The listing builds one solid part. Answer for the finished solid, in the listing's coordinates (mm). A direction names the side the tool comes from. Round coordinates to 2 decimals unless told otherwise and drop trailing zeros. Write each loop counter-clockwise with the first axis right and the second up, starting at its lowest first coordinate (ties: lowest second). Pieces come first, ordered by that corner, then holes. Notation, with made-up numbers: M 82.5,-3 L 135.5,-3 A16 cw 135.5,21 Z; hole C 13.5,38 d6. An arc over 180 degrees is marked long. Put each result on its own line as item: value. Start each with the question number.
Autodesk Inventor part; units mm, degrees
ref_plane "YZ Plane" through (0, 0, 0) normal (1, 0, 0) x (0, 1, 0)
ref_plane "XZ Plane" through (0, 0, 0) normal (0, 1, 0) x (-1, 0, 0)
ref_plane "XY Plane" through (0, 0, 0) normal (0, 0, 1) x (1, 0, 0)
sketch "Sketch9" plane through (0, 0, 0) normal (0, 1, 0) x (-1, 0, 0)
  line L0 (15, 15) -> (-15, 15)
  line L1 (-15, 15) -> (-15, -15)
  line L2 (-15, -15) -> (15, -15)
  line L3 (15, -15) -> (15, 15)
  line L4 (15, 15) -> (-15, -15) construction
  line L5 (-15, 15) -> (15, -15) construction
  line L6 (-13, 13) -> (13, 13)
  line L7 (13, 13) -> (13, -13)
  line L8 (13, -13) -> (-13, -13)
  line L9 (-13, -13) -> (-13, 13)
  point P0 (0, 0)
  dimension "d172" = 30
  dimension "d173" = 30
  dimension "d174" = 2
extrude "Extrusion3" add sketch "Sketch9" against normal blind 250
sketch "Sketch10" plane through (0, 0, 0) normal (1, 0, 0) x (0, 1, 0)
  line L0 (0, 15) -> (0, -15) construction
  line L1 (0, 15) -> (-250, 15) construction
  line L2 (0, -15) -> (-250, -15) construction
  line L3 (-58.5, 8.5) -> (-41.5, 8.5)
  line L4 (-41.5, 8.5) -> (-41.5, -8.5)
  line L5 (-41.5, -8.5) -> (-58.5, -8.5)
  line L6 (-58.5, -8.5) -> (-58.5, 8.5)
  line L7 (-58.5, 8.5) -> (-41.5, -8.5) construction
  line L8 (-41.5, 8.5) -> (-58.5, -8.5) construction
  line L9 (0, 0) -> (30, 0)
  circle A0 centre (-50, 0) radius 8.5
  dimension "d177" = 17
  dimension "d178" = 17
  dimension "d181" = 30
  dimension "d182" = 80
extrude "Extrusion4" cut sketch "Sketch10" along normal through all contours A0
pattern_linear "Rectangular Pattern4" count 4 spacing 68 along (0, -1, 0) of "Extrusion4"
properties part number "PRS 1662 FDS 1000 way tube 4_D940" material "Stainless Steel"
Item 1: Section D-D (y = -118) is taken. Give the vertices of the cut face in (x, z), and give its area (3 significant figures).
Item 2: Section B-B (z = 0) is taken. Give the vertices of the cut face in (x, y), and give its area (3 significant figures).
Item 3: Section A-A (x = 3.5) is taken. Give the vertices of the cut face in (y, z).
Item 4: Which of the six approach directions +Z, -Z, +X, -X, +Y, -Y give full straight-line access (tool end or side, diameter ignored) to faces 4 (the flat face through (-13.3, -250, -1)), 5 (the flat face through (0, -123, -13)), 6 (the cylindrical face through (13.99, -109.89, -2.55))?
Item 5: Section C-C (y = -68) is taken. Give the vertices of the cut face in (x, z), and give its area (3 significant figures).
Item 6: A flat-ended cylindrical pin translates along its axis: pin 1 (13.5 mm diameter, centred on y = -118, z = 0, fed in from +X). Find the tip coordinate at first contact, or state that the pin passes through.
Item 7: Determine the mould class of faces 1 (the cylindrical face through (14, -245.5, 0.1)), 2 (the flat face through (15, -123.3, 6.9)), 3 (the flat face through (0, -123, 15)) for opening direction Z: released by +Z, released by -Z, zero draft, split by the parting line, or undercut.
Item 8: Consider line 1 along Y through (x, z) = (14.3, 0); line 2 along Z through (x, y) = (14.6, -50); line 3 along Z through (x, y) = (-8.5, -231.5). Determine where each line is inside the solid, lowest interval first. Write a range as [from, to].
Output values:
1. outline: M -15,-15 L 15,-15 L 15,-8.5 L 13,-8.5 L 13,-13 L -13,-13 L -13,13 L 13,13 L 13,8.5 L 15,8.5 L 15,15 L -15,15 Z
1. area: 190 mm^2
2. outline: M -15,-250 L -13,-250 L -13,0 L -15,0 Z; M 13,-245.5 L 15,-245.5 L 15,-194.5 L 13,-194.5 Z; M 13,-177.5 L 15,-177.5 L 15,-126.5 L 13,-126.5 Z; M 13,-109.5 L 15,-109.5 L 15,-58.5 L 13,-58.5 Z; M 13,-41.5 L 15,-41.5 L 15,0 L 13,0 Z
2. area: 889 mm^2
3. outline: M -250,-15 L 0,-15 L 0,-13 L -250,-13 Z; M -250,13 L 0,13 L 0,15 L -250,15 Z
4. face 4: +Z, -Z, +X, -X, -Y
4. face 5: +Y, -Y
4. face 6: +X
5. outline: M -15,-15 L 15,-15 L 15,15 L -15,15 Z; hole M -13,-13 L 13,-13 L 13,13 L -13,13 Z
5. area: 224 mm^2
6. pin 1: stops at x = -13
7. face 1: undercut
7. face 2: zero draft
7. face 3: released by +Z
8. line 1: y = [-245.5, -194.5], [-177.5, -126.5], [-109.5, -58.5], [-41.5, 0]
8. line 2: z = [-15, -8.5], [8.5, 15]
8. line 3: z = [-15, -13], [13, 15]
